from build123d import *

# Parameters (mm, degrees)
SKETCH1_W           = 40
SKETCH1_H           = 40
SKETCH1_R           = 4
BOSS_EXTRUDE1_DEPTH = 5
SKETCH2_W           = 40
SKETCH2_H           = 40
SKETCH2_R           = 4
BOSS_EXTRUDE2_DEPTH = 5


with BuildPart() as part:
    # Sketch1 → Boss-Extrude1 (new body)
    with BuildSketch(Plane(origin=(0, 0, 0), x_dir=(1, 0, 0), z_dir=(0, 1, 0))):
        Rectangle(SKETCH1_W, SKETCH1_H)
        with Locations(Location((0, 0, 0), (0, 0, 270))):
            Circle(SKETCH1_R, mode=Mode.SUBTRACT)
    extrude(amount=BOSS_EXTRUDE1_DEPTH)

    # Sketch2 → Boss-Extrude2 (add)
    with BuildSketch(Plane(origin=(20, 0, 0), x_dir=(0, 0, -1), z_dir=(1, 0, 0))):
        with Locations((0, 20)):
            Rectangle(SKETCH2_W, SKETCH2_H)
        with Locations((0, 20)):
            Circle(SKETCH2_R, mode=Mode.SUBTRACT)
    extrude(amount=BOSS_EXTRUDE2_DEPTH)


solid = part.part
The model under review builds one solid part; all positions refer to its coordinate system, in mm. A direction names the side the tool comes from. Coordinates: 2 decimals unless noted, no trailing zeros. Loops run counter-clockwise (first coordinate to the right, second up) from the corner with the lowest first, then second, coordinate; pieces in that order, holes last. Notation, with made-up numbers: M 11,-17.75 L 59,-17.75 A30 ccw 59,21.25 Z; hole C 6,78 d1. An arc over 180 degrees is marked long. Put each result on its own line as item: value. Start each with the question number.
Q1. Add section D-D (z = -6.5). Write out the cut boundary in (x, y), and give its area (3 significant figures).
Q2. Wall thickness on line 1 (X direction, y = 1.4, z = 0); line 2 (Y direction, x = 23.55, z = 0); line 3 (X direction, y = 28, z = 2): over which ranges is each line inside the solid? List them lowest first.
Q3. Add section C-C (z = 0). Write out the cut boundary in (x, y), and give its area (3 significant figures).
Q4. Add section A-A (y = 20). Write out the cut boundary in (x, z).
Q5. Clearance check with a flat-ended pin moving along its axis: pin 1 (12 mm diameter, centred on x = -1, z = -3.5, fed in from +Y). State where the tip first meets the part, or that it passes through.
Q6. For faces 4 (the flat face through (2, 0, -4)), 5 (the flat face through (20, 27, 0)), list the 3-axis set-ups (+Z, -Z, +X, -X, +Y, -Y) from which the entire face can be reached by the end or side of a thin tool; tool diameter is ignored.
Q7. The part is to be moulded in two halves that separate along Z. For faces 1 (the flat face through (12, 4, 20)), 2 (the flat face through (-20, 2, 0)), 3 (the cylindrical face through (-3.905, 2.465, -0.867)), say which applies: +Z half, -Z half, draft (parallel to the pull), parting line (faces both ways), or undercut.
Q8. Add section B-B (x = 0). Write out the cut boundary in (y, z), and give its area (3 significant figures).
Answers:
1. outline: M -20,0 L 25,0 L 25,40 L 20,40 L 20,5 L -20,5 Z
1. area: 400 mm^2
2. line 1: x = -20 to -4, 4 to 25
2. line 2: y = 0 to 16, 24 to 40
2. line 3: x = 20 to 25
3. outline: M -20,0 L -4,0 L -4,5 L -20,5 Z; M 4,0 L 25,0 L 25,16 L 20,16 L 20,5 L 4,5 Z; M 20,24 L 25,24 L 25,40 L 20,40 Z
3. area: 320 mm^2
4. outline: M 20,-20 L 25,-20 L 25,-4 L 20,-4 Z; M 20,4 L 25,4 L 25,20 L 20,20 Z
5. pin 1: stops at y = 5
6. face 4: +Z, -Z, +X, -X, -Y
6. face 5: +Z, -Z, -X, +Y
7. face 1: +Z half
7. face 2: draft
7. face 3: undercut
8. outline: M 0,-20 L 5,-20 L 5,-4 L 0,-4 Z; M 0,4 L 5,4 L 5,20 L 0,20 Z
8. area: 160 mm^2
